Can you work these out from the model? Positions are in its coordinate system, mm. Face numbers are marked on the shaded views. A direction names the side the tool comes from. Coordinates: 2 decimals unless noted, no trailing zeros. Order: outer loops, then holes, each group sorted by start corner. A loop starts at its lowest first (then second) coordinate and runs counter-clockwise, first axis right, second up. Notation, with made-up numbers: (21, -11.5) -> (39, -11.5) arc R10 ccw to (39, -4.5) -> close; hole circle Ø6 at (-28.75, 44.5). An arc over 180 degrees is marked (long way). Write item = value, one per line. Start each with the question number.
from build123d import *

# Parameters (mm, degrees)
M12_TAPPED_HOLE1_D           = 10.2
M12_TAPPED_HOLE1_DEPTH       = 15
M12_TAPPED_HOLE1_CSINK_D     = 12.05
M12_TAPPED_HOLE1_CSINK_ANGLE = 90
M12_TAPPED_HOLE1_TIP         = 3.064389157
M12_TAPPED_HOLE3_D           = 10.2
M12_TAPPED_HOLE3_DEPTH       = 15
M12_TAPPED_HOLE3_CSINK_D     = 12.05
M12_TAPPED_HOLE3_CSINK_ANGLE = 90
M12_TAPPED_HOLE3_TIP         = 3.064389157
M24_TAPPED_HOLE2_D           = 21
M24_TAPPED_HOLE2_DEPTH       = 33
M24_TAPPED_HOLE2_CSINK_D     = 24.05
M24_TAPPED_HOLE2_CSINK_ANGLE = 90
M24_TAPPED_HOLE2_TIP         = 6.3090365
CUT_EXTRUDE1_REACH           = 211.077
SKETCH3_R                    = 10


with BuildPart() as part:
    # Sketch2 → Revolve1 (revolve)
    with BuildSketch(Plane.XY, mode=Mode.PRIVATE) as revolve1_sk:
        with BuildLine():
            Line((7, 0), (7, 20.875644347))
            Line((7, 20.875644347), (28, 33))
            Line((28, 33), (28, 81))
            Line((28, 81), (88, 81))
            ThreePointArc((88, 81), (89.757359313, 76.757359313), (94, 75))
            Line((94, 75), (138, 75))
            Line((138, 75), (138, 53))
            Line((138, 53), (81, 53))
            Line((81, 53), (81, 47))
            Line((81, 47), (35, 0))
            Line((35, 0), (7, 0))
        make_face()
    revolve(revolve1_sk.sketch.rotate(Axis((0, 0, 0), (0, 1, 0)), 90), axis=Axis((0, 0, 0), (0, 1, 0)))

    # M12 Tapped Hole1
    with Locations(Plane(origin=(0, 81, 0), x_dir=(1, 0, 0), z_dir=(0, 1, 0))):
        with Locations((0.035531834, -44.277728927)):
            CounterSinkHole(M12_TAPPED_HOLE1_D / 2, M12_TAPPED_HOLE1_CSINK_D / 2, depth=M12_TAPPED_HOLE1_DEPTH, counter_sink_angle=M12_TAPPED_HOLE1_CSINK_ANGLE)
            with Locations((0, 0, -(M12_TAPPED_HOLE1_DEPTH + M12_TAPPED_HOLE1_TIP / 2))):  # 118° drill point
                Cone(0, M12_TAPPED_HOLE1_D / 2, M12_TAPPED_HOLE1_TIP, mode=Mode.SUBTRACT)

    # M12 Tapped Hole3
    with Locations(Plane(origin=(0, 81, 0), x_dir=(1, 0, 0), z_dir=(0, 1, 0))):
        with Locations((0, 44)):
            CounterSinkHole(M12_TAPPED_HOLE3_D / 2, M12_TAPPED_HOLE3_CSINK_D / 2, depth=M12_TAPPED_HOLE3_DEPTH, counter_sink_angle=M12_TAPPED_HOLE3_CSINK_ANGLE)
            with Locations((0, 0, -(M12_TAPPED_HOLE3_DEPTH + M12_TAPPED_HOLE3_TIP / 2))):  # 118° drill point
                Cone(0, M12_TAPPED_HOLE3_D / 2, M12_TAPPED_HOLE3_TIP, mode=Mode.SUBTRACT)

    # M24 Tapped Hole2
    with Locations(Plane(origin=(0, 81, 0), x_dir=(1, 0, 0), z_dir=(0, 1, 0))):
        with Locations((59.673816791, 0.403201465), (0, 0), (-60.480219721, 0.80640293)):
            CounterSinkHole(M24_TAPPED_HOLE2_D / 2, M24_TAPPED_HOLE2_CSINK_D / 2, depth=M24_TAPPED_HOLE2_DEPTH, counter_sink_angle=M24_TAPPED_HOLE2_CSINK_ANGLE)
            with Locations((0, 0, -(M24_TAPPED_HOLE2_DEPTH + M24_TAPPED_HOLE2_TIP / 2))):  # 118° drill point
                Cone(0, M24_TAPPED_HOLE2_D / 2, M24_TAPPED_HOLE2_TIP, mode=Mode.SUBTRACT)

    # Sketch3 → Cut-Extrude1 (cut, up to next)
    with BuildSketch(Plane(origin=(0, 75, 0), x_dir=(1, 0, 0), z_dir=(0, 1, 0)), mode=Mode.PRIVATE) as cut_extrude1_sk1:
        with Locations(Location((0, 112.5, 0), (0, 0, 270))):
            Circle(SKETCH3_R)
    cut_extrude1_tool1 = extrude(cut_extrude1_sk1.sketch, amount=-CUT_EXTRUDE1_REACH, mode=Mode.PRIVATE) & part.part
    # Sketch3 → Cut-Extrude1 (cut, up to next)
    with BuildSketch(Plane(origin=(0, 75, 0), x_dir=(1, 0, 0), z_dir=(0, 1, 0)), mode=Mode.PRIVATE) as cut_extrude1_sk2:
        with Locations(Location((97.427857926, 56.25, 0), (0, 0, 270))):
            Circle(SKETCH3_R)
    cut_extrude1_tool2 = extrude(cut_extrude1_sk2.sketch, amount=-CUT_EXTRUDE1_REACH, mode=Mode.PRIVATE) & part.part
    # Sketch3 → Cut-Extrude1 (cut, up to next)
    with BuildSketch(Plane(origin=(0, 75, 0), x_dir=(1, 0, 0), z_dir=(0, 1, 0)), mode=Mode.PRIVATE) as cut_extrude1_sk3:
        with Locations(Location((97.427857926, -56.25, 0), (0, 0, 270))):
            Circle(SKETCH3_R)
    cut_extrude1_tool3 = extrude(cut_extrude1_sk3.sketch, amount=-CUT_EXTRUDE1_REACH, mode=Mode.PRIVATE) & part.part
    # Sketch3 → Cut-Extrude1 (cut, up to next)
    with BuildSketch(Plane(origin=(0, 75, 0), x_dir=(1, 0, 0), z_dir=(0, 1, 0)), mode=Mode.PRIVATE) as cut_extrude1_sk4:
        with Locations(Location((0, -112.5, 0), (0, 0, 270))):
            Circle(SKETCH3_R)
    cut_extrude1_tool4 = extrude(cut_extrude1_sk4.sketch, amount=-CUT_EXTRUDE1_REACH, mode=Mode.PRIVATE) & part.part
    # Sketch3 → Cut-Extrude1 (cut, up to next)
    with BuildSketch(Plane(origin=(0, 75, 0), x_dir=(1, 0, 0), z_dir=(0, 1, 0)), mode=Mode.PRIVATE) as cut_extrude1_sk5:
        with Locations(Location((-97.427857926, -56.25, 0), (0, 0, 270))):
            Circle(SKETCH3_R)
    cut_extrude1_tool5 = extrude(cut_extrude1_sk5.sketch, amount=-CUT_EXTRUDE1_REACH, mode=Mode.PRIVATE) & part.part
    # Sketch3 → Cut-Extrude1 (cut, up to next)
    with BuildSketch(Plane(origin=(0, 75, 0), x_dir=(1, 0, 0), z_dir=(0, 1, 0)), mode=Mode.PRIVATE) as cut_extrude1_sk6:
        with Locations(Location((-97.427857926, 56.25, 0), (0, 0, 270))):
            Circle(SKETCH3_R)
    cut_extrude1_tool6 = extrude(cut_extrude1_sk6.sketch, amount=-CUT_EXTRUDE1_REACH, mode=Mode.PRIVATE) & part.part
    add(cut_extrude1_tool1.solids().sort_by_distance((0, 75, -112.5))[0], mode=Mode.SUBTRACT)
    add(cut_extrude1_tool2.solids().sort_by_distance((97.427858, 75, -56.25))[0], mode=Mode.SUBTRACT)
    add(cut_extrude1_tool3.solids().sort_by_distance((97.427858, 75, 56.25))[0], mode=Mode.SUBTRACT)
    add(cut_extrude1_tool4.solids().sort_by_distance((0, 75, 112.5))[0], mode=Mode.SUBTRACT)
    add(cut_extrude1_tool5.solids().sort_by_distance((-97.427858, 75, 56.25))[0], mode=Mode.SUBTRACT)
    add(cut_extrude1_tool6.solids().sort_by_distance((-97.427858, 75, -56.25))[0], mode=Mode.SUBTRACT)


solid = part.part
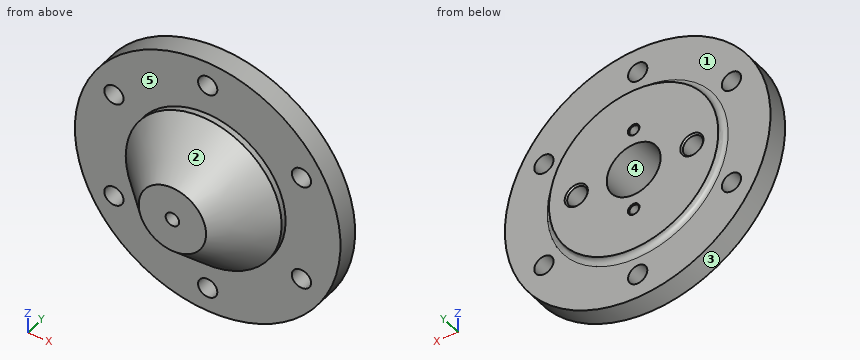
(1) Imagine slicing it at B-B (z = 57.5). Count the separate pieces of the cut face and the enclosed holes in it, plus the area to 3 significant figures.
(2) Imagine slicing it at C-C (x = -111.5). Write out the boundary of the cut face in (y, z).
(3) If I drill on L1, parallel to Y at x = 121.5, z = 26; L2, parallel to X at y = 14.5, z = 0.5; L3, parallel to X at y = 66, z = -56.25, over which ranges is the centre line in solid material (lowest first)? Write a range as from..to.
(4) For P1, Ø12, axis at x = -97.43, z = -56.25, coming from the +Y side; P2, Ø1, axis at x = 34.5, y = 14.5, coming from the +Z side; P3, Ø19, axis at x = 59.67, z = -0.4, coming from the +Y side; P4, Ø12.5, axis at x = -60.48, z = -0.81, coming from the +Y side, each with a flat end and sliding along its axis, tell me the tip position at first contact or that it passes through.
(5) For the marked faces 1 and 2, which set-ups out of +Z, -Z, +X, -X, +Y, -Y let a thin tool reach every point of the face, with its end or its side?
(6) Imagine slicing it at D-D (z = 112.5). Write out the boundary of the cut face in (x, y), plus the area to 3 significant figures.
(7) Imagine slicing it at A-A (z = -111). Write out the boundary of the cut face in (x, y).
(8) Thinking about a two-plate mould opening in Z: for the marked faces 3, 4 and 5, which applies, +Z half, -Z half, draft (parallel to the pull), parting line (faces both ways), or undercut?
Result set:
q1.separate_pieces = 3
q1.enclosed_holes = 0
q1.area = 7,910 mm2
q2.outline = (53, -81.31) -> (75, -81.31) -> (75, 81.31) -> (53, 81.31) -> close
q3.L1 = 53..75
q3.L2 = -49.19..-6.98, 6.98..49.19
q3.L3 = -126.02..-107.43, -87.43..87.43, 107.43..126.02
q4.P1 = through
q4.P2 = 35.9
q4.P3 = 47.4
q4.P4 = 45.45
q5.face_1 = +Y
q5.face_2 = -Y
q6.outline = (-79.92, 53) -> (-10, 53) -> (-10, 75) -> (-79.92, 75) -> close; (10, 53) -> (79.92, 53) -> (79.92, 75) -> (10, 75) -> close
q6.area = 3,080 mm2
q7.outline = (-81.99, 53) -> (-9.89, 53) -> (-9.89, 75) -> (-81.99, 75) -> close; (9.89, 53) -> (81.99, 53) -> (81.99, 75) -> (9.89, 75) -> close
q8.face_3 = parting line
q8.face_4 = undercut
q8.face_5 = draft
